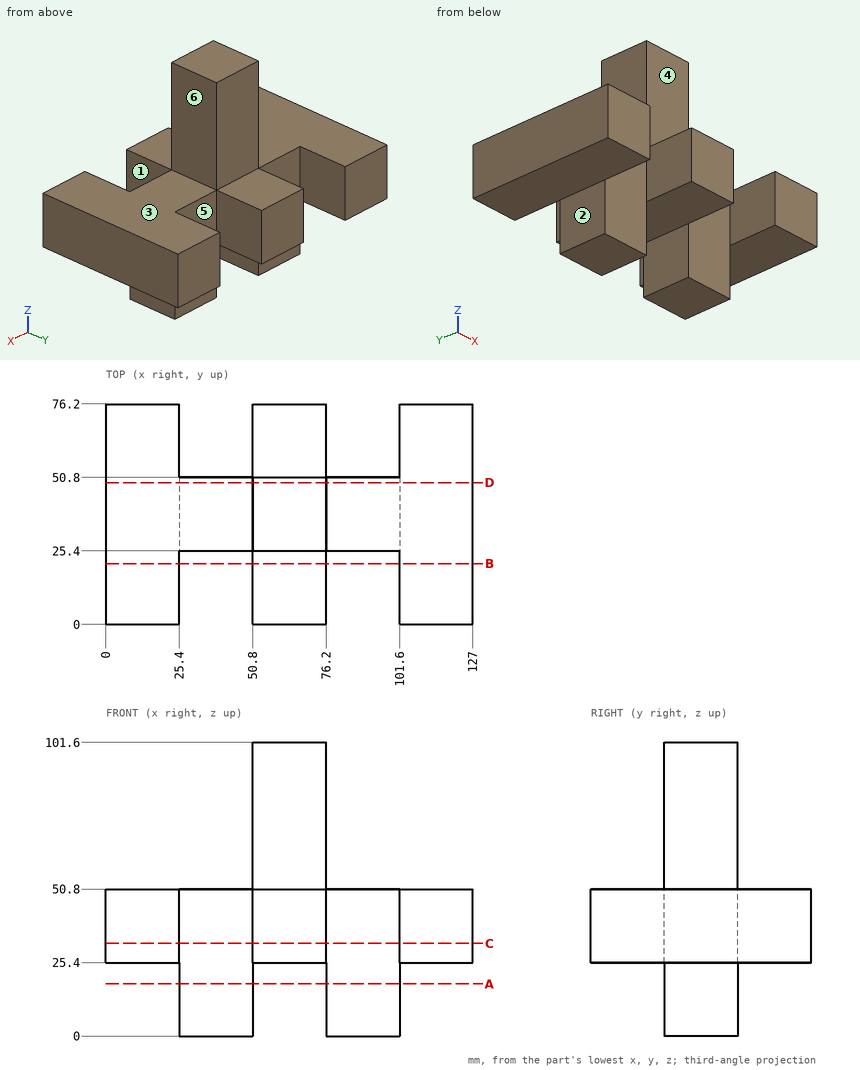
Verification items for this drawing (mm, ordinates from the low corner). A direction names the side the tool comes from. Coordinates: 2 decimals unless noted, no trailing zeros. Loops run counter-clockwise (first coordinate to the right, second up) from the corner with the lowest first, then second, coordinate; pieces in that order, holes last.
Item 1: Sectioned sample at C-C, the plane z = 32. Record the boundary of the cut face in (x, y).
Item 2: Sectioned sample at B-B, the plane y = 21. Record the boundary of the cut face in (x, z), then the cut area to 3 significant figures.
Item 3: Access from +Z, -Z, +X, -X, +Y, -Y to the whole of each face (thin tool, end or side, straight path). Record for the marked faces 4, 5 and 6.
Item 4: Go/stop test with flat-tipped pins: pin 1 Ø12.5 at (y, z) = (37.5, 12) entering from +X; pin 2 Ø12 at (y, z) = (55, 90.5) entering from +X; pin 3 Ø7.5 at (x, z) = (88, 25) entering from -Y; pin 4 Ø20.5 at (x, z) = (93, 22) entering from +Y. Record where each tip stops, or that it passes through.
Item 5: Sectioned sample at A-A, the plane z = 18. Record the boundary of the cut face in (x, y).
Item 6: Thickness scan on line 1 (X direction, y = 60, z = 36); line 2 (X direction, y = 47.5, z = 7.5); line 3 (Z direction, x = 67.5, y = 11). Record the ranges inside material, lowest first.
Item 7: Sectioned sample at D-D, the plane y = 49. Record the boundary of the cut face in (x, z), then the cut area to 3 significant figures.
Item 8: Release check for a two-part mould opening along X. For the marked faces 1, 2 and 3 record: released by +X, released by -X, zero draft, split by the parting line, or undercut.
Check result:
1. outline: (0, 0) - (25.4, 0) - (25.4, 25.4) - (50.8, 25.4) - (50.8, 0) - (76.2, 0) - (76.2, 25.4) - (101.6, 25.4) - (101.6, 0) - (127, 0) - (127, 76.2) - (101.6, 76.2) - (101.6, 50.8) - (76.2, 50.8) - (76.2, 76.2) - (50.8, 76.2) - (50.8, 50.8) - (25.4, 50.8) - (25.4, 76.2) - (0, 76.2) - close
2. outline: (0, 25.4) - (25.4, 25.4) - (25.4, 50.8) - (0, 50.8) - close; (50.8, 25.4) - (76.2, 25.4) - (76.2, 50.8) - (50.8, 50.8) - close; (101.6, 25.4) - (127, 25.4) - (127, 50.8) - (101.6, 50.8) - close
2. area: 1,940 mm2
3. face 4: +Z, +X, -X, -Y
3. face 5: +Z, -Z, +Y
3. face 6: +Z, +X, +Y, -Y
4. pin 1: stops at x = 101.6
4. pin 2: stops at x = 76.2
4. pin 3: stops at y = 25.4
4. pin 4: stops at y = 76.2
5. outline: (25.4, 25.4) - (50.8, 25.4) - (50.8, 50.8) - (25.4, 50.8) - close; (76.2, 25.4) - (101.6, 25.4) - (101.6, 50.8) - (76.2, 50.8) - close
6. line 1: x = 0 to 25.4, 50.8 to 76.2, 101.6 to 127
6. line 2: x = 25.4 to 50.8, 76.2 to 101.6
6. line 3: z = 25.4 to 50.8
7. outline: (0, 25.4) - (25.4, 25.4) - (25.4, 0) - (50.8, 0) - (50.8, 25.4) - (76.2, 25.4) - (76.2, 0) - (101.6, 0) - (101.6, 25.4) - (127, 25.4) - (127, 50.8) - (76.2, 50.8) - (76.2, 101.6) - (50.8, 101.6) - (50.8, 50.8) - (0, 50.8) - close
7. area: 5,810 mm2
8. face 1: undercut
8. face 2: released by -X
8. face 3: zero draft
